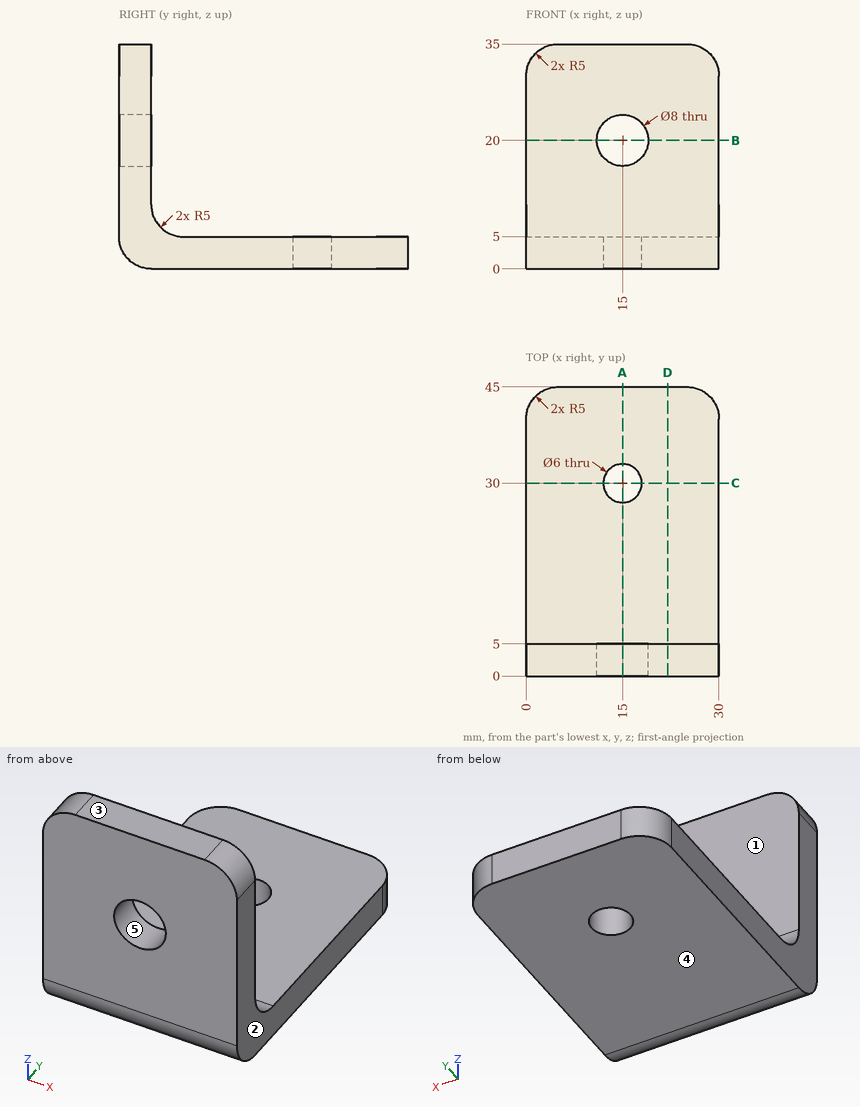
Could you check a few things on this drawing? It's one solid part, dimensions in mm from its lowest x, y, z. A direction names the side the tool comes from. Give positions to 0.01 mm unless a question says otherwise; leave off trailing zeros. Order: outer loops, then holes, each group sorted by start corner. A loop starts at its lowest first (then second) coordinate and runs counter-clockwise, first axis right, second up. Notation, with made-up numbers: (86, 1) -> (120, 1) arc R17 ccw to (120, 16) -> close; hole circle Ø6 at (53, 37.25). An arc over 180 degrees is marked (long way). Use CSV: the item, a comma, the result in double quotes. Start each with the question number.
Item 1: Suppose I cut it at C-C (y = 30). List the corners of the cut face in (x, z) for me, and give its area (3 significant figures).
Item 2: If I drill on probe 1 along Z at (x, y) = (25, 33); probe 2 along X at (y, z) = (2.25, 20), over which ranges is the centre line in solid material (lowest first)? Write a range as [from, to].
Item 3: Thinking about a two-plate mould opening in Z: for the marked faces 3, 4 and 5, which applies, pulls with the +Z half, pulls with the -Z half, needs draft (parallel to the pull), parting line crosses it, or undercut?
Item 4: Suppose I cut it at A-A (x = 15). List the corners of the cut face in (y, z) for me.
Item 5: Suppose I cut it at D-D (x = 22). List the corners of the cut face in (y, z) for me.
Item 6: I'm going to push flat-ended pins straight in: P1, Ø9, axis at x = 15, z = 20, coming from the +Y side; P2, Ø3, axis at x = 13, z = 10.5, coming from the +Y side; P3, Ø9, axis at x = 20.5, y = 29.5, coming from the +Z side. Where does each tip first touch, or does it pass through?
Item 7: Suppose I cut it at B-B (z = 20). List the corners of the cut face in (x, y) for me, and give its area (3 significant figures).
Item 8: On a 3-axis mill with a long thin cutter (end or side, diameter ignored), from which of +Z, -Z, +X, -X, +Y, -Y can I reach the whole of each face in a straight line? I mean the marked faces 1 and 2. Say none if no direction works.
Answer block:
1,outline,"(0, 0) -> (12, 0) -> (12, 5) -> (0, 5) -> close; (18, 0) -> (30, 0) -> (30, 5) -> (18, 5) -> close"
1,area,"120 mm^2"
2,probe 1,"z = [0, 5]"
2,probe 2,"x = [0, 11], [19, 30]"
3,face 3,"pulls with the +Z half"
3,face 4,"pulls with the -Z half"
3,face 5,"undercut"
4,outline,"(0, 5) arc R5 ccw to (5, 0) -> (27, 0) -> (27, 5) -> (10, 5) arc R5 cw to (5, 10) -> (5, 16) -> (0, 16) -> close; (0, 24) -> (5, 24) -> (5, 35) -> (0, 35) -> close; (33, 0) -> (45, 0) -> (45, 5) -> (33, 5) -> close"
5,outline,"(0, 5) arc R5 ccw to (5, 0) -> (45, 0) -> (45, 5) -> (10, 5) arc R5 cw to (5, 10) -> (5, 35) -> (0, 35) -> close"
6,P1,"stops at y = 5"
6,P2,"stops at y = 5.1"
6,P3,"stops at z = 5"
7,outline,"(0, 0) -> (11, 0) -> (11, 5) -> (0, 5) -> close; (19, 0) -> (30, 0) -> (30, 5) -> (19, 5) -> close"
7,area,"110 mm^2"
8,face 1,"+Z, +X, -X, +Y"
8,face 2,"+Z, -Z, +X, +Y, -Y"
